Model file for the job. Use its own axes, mm. Round coordinates to 2 decimals unless told otherwise and drop trailing zeros. Loops run counter-clockwise (first coordinate to the right, second up) from the corner with the lowest first, then second, coordinate; pieces in that order, holes last. Notation, with made-up numbers: M 73,19 L 122,19 A30 cw 122,54 Z; hole C -23,6 d6. An arc over 180 degrees is marked long. Use a Markdown table: item, result. Add a question column.
Q1. Pin check, flat tip, straight feed: pin 1 (3 mm diameter, centred on x = -13.44, y = 25.4, fed in from +Z). Stop position of the tip, or through.
Q2. Cut at C-C (y = -26). Give the cut face in (x, z).
Q3. Cut at B-B (y = 25.4). Give the cut face in (x, z).
Q4. Cut at A-A (z = 0.75). Give the cut face in (x, y), plus the area to 3 significant figures.
Q5. Cut at D-D (x = 0). Give the cut face in (y, z).
Q6. Probe line 1 (X direction, y = -23.5, z = 0.8); line 2 (X direction, y = 24.5, z = 1.2); line 3 (Y direction, x = 0, z = 1.3). List the from-to ranges inside material, lowest first. Write a range as from..to.
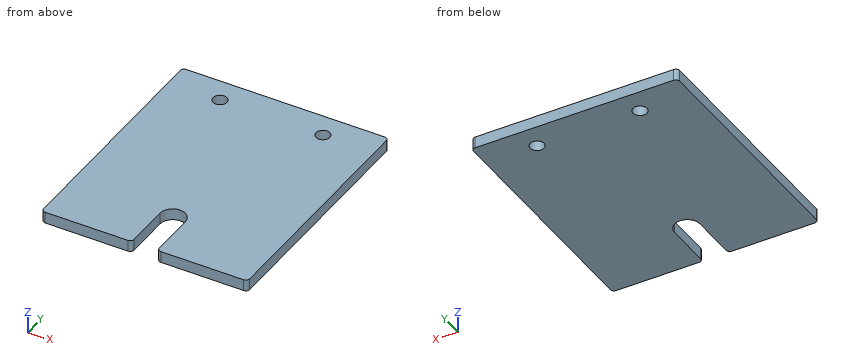
from build123d import *

# Parameters (mm, degrees)
SKETCH_R  = 1.8288
PAD_DEPTH = 3


with BuildPart() as part:
    # Sketch → Pad (new body)
    with BuildSketch(Plane.XY):
        with BuildLine():
            ThreePointArc((-25.9, 31.75), (-26.607107, 31.457107), (-26.9, 30.75))
            Line((-26.9, -30.75), (-26.9, 30.75))
            ThreePointArc((-26.9, -30.75), (-26.607107, -31.457107), (-25.9, -31.75))
            Line((-25.9, -31.75), (-4.302, -31.75))
            ThreePointArc((-4.302, -31.75), (-3.594893, -31.457107), (-3.302, -30.75))
            Line((-3.302, -19.05), (-3.302, -30.75))
            ThreePointArc((3.302, -19.05), (0, -15.748), (-3.302, -19.05))
            Line((3.302, -19.05), (3.302, -30.75))
            ThreePointArc((3.302, -30.75), (3.594893, -31.457107), (4.302, -31.75))
            Line((4.302, -31.75), (25.9, -31.75))
            ThreePointArc((25.9, -31.75), (26.607107, -31.457107), (26.9, -30.75))
            Line((26.9, 30.75), (26.9, -30.75))
            ThreePointArc((26.9, 30.75), (26.607107, 31.457107), (25.9, 31.75))
            Line((-25.9, 31.75), (25.9, 31.75))
        make_face()
        with Locations((-13.4352, 25.4)):
            Circle(SKETCH_R, mode=Mode.SUBTRACT)
        with Locations((13.4352, 25.4)):
            Circle(SKETCH_R, mode=Mode.SUBTRACT)
    extrude(amount=PAD_DEPTH)


solid = part.part
Checked values:
| question | item | result |
|---|---|---|
| 1 | pin 1 | passes through |
| 2 | outline | M -26.9,0 L -3.3,0 L -3.3,3 L -26.9,3 Z; M 3.3,0 L 26.9,0 L 26.9,3 L 3.3,3 Z |
| 3 | outline | M -26.9,0 L -15.26,0 L -15.26,3 L -26.9,3 Z; M -11.61,0 L 11.61,0 L 11.61,3 L -11.61,3 Z; M 15.26,0 L 26.9,0 L 26.9,3 L 15.26,3 Z |
| 4 | outline | M -26.9,-30.75 A1 ccw -25.9,-31.75 L -4.3,-31.75 A1 ccw -3.3,-30.75 L -3.3,-19.05 A3.3 cw 3.3,-19.05 L 3.3,-30.75 A1 ccw 4.3,-31.75 L 25.9,-31.75 A1 ccw 26.9,-30.75 L 26.9,30.75 A1 ccw 25.9,31.75 L -25.9,31.75 A1 ccw -26.9,30.75 Z; hole C -13.44,25.4 d3.66; hole C 13.44,25.4 d3.66 |
| 4 | area | 3,290 mm^2 |
| 5 | outline | M -15.75,0 L 31.75,0 L 31.75,3 L -15.75,3 Z |
| 6 | line 1 | x = -26.9..-3.3, 3.3..26.9 |
| 6 | line 2 | x = -26.9..-15.03, -11.84..11.84, 15.03..26.9 |
| 6 | line 3 | y = -15.75..31.75 |
